```python
from build123d import *

# Parameters (mm, degrees)
F2_W       = 140
F2_H       = 140
F3_DEPTH   = 500
F4_SIZE2   = 100
F4_SIZE    = 40
F4_2_SIZE2 = 100
F4_2_SIZE  = 40
F6_DEPTH   = 70
F7_W       = 60
F7_H       = 40
F8_DEPTH   = 60


with BuildPart() as f3:
    # F2 (on Front) → F3 (new body, symmetric)
    with BuildSketch(Plane.XZ):
        Rectangle(F2_W, F2_H)
    extrude(amount=F3_DEPTH, both=True)

    # F4
    f4_edges = [f3.edges().sort_by_distance(p)[0] for p in [
        (0, -500, 70),
    ]]
    f4_side = f3.faces().sort_by_distance((0, -500, 0))[0]
    chamfer(f4_edges, length=F4_SIZE, length2=F4_SIZE2, reference=f4_side)

    # F4#2
    f4_2_edges = [f3.edges().sort_by_distance(p)[0] for p in [
        (0, 500, 70),
    ]]
    f4_2_side = f3.faces().sort_by_distance((0, 500, 0))[0]
    chamfer(f4_2_edges, length=F4_2_SIZE, length2=F4_2_SIZE2, reference=f4_2_side)

    # F5 (on Right) → F6 (cut, symmetric)
    with BuildSketch(Plane.YZ):
        Polygon((200, -30), (0, -30), (-200, -30), (-300, -70), (0, -70), (300, -70), align=None)
    extrude(amount=F6_DEPTH, both=True, mode=Mode.SUBTRACT)

    # F7 (on face) → F8 (cut)
    with BuildSketch(Plane.XY.offset(70)):
        with Locations((0, -325)):
            Rectangle(F7_W, F7_H)
        with Locations((0, 225)):
            Rectangle(F7_W, F7_H)
    extrude(amount=-F8_DEPTH, mode=Mode.SUBTRACT)


solid = f3.part
```
Design review of the part built by this model. Coordinates are the model's own, in mm. A direction names the side the tool comes from. Coordinates: 2 decimals unless noted, no trailing zeros. Order: outer loops, then holes, each group sorted by start corner. A loop starts at its lowest first (then second) coordinate and runs counter-clockwise, first axis right, second up. Notation, with made-up numbers: M -35.75,75.25 L -20.75,75.25 A22 cw -20.75,92.25 Z; hole C -33.75,88 d1. An arc over 180 degrees is marked long. Answer as a JSON object with one key per item and string values. Group by question number.
1) Wall thickness on L1, parallel to Y at x = -21.5, z = 20; L2, parallel to Z at x = 33, y = 22; L3, parallel to Y at x = -45, z = -59: over which ranges is each line inside the solid? List them lowest first.
2) For pin 1 (3 mm diameter, centred on x = 44.5, z = 51, fed in from +Y); pin 2 (1.5 mm diameter, centred on x = 9, z = 55, fed in from +Y) (3 decimals), all flat-tipped, find the tip position at first contact; note any pin that passes through.
3) Add section D-D, the plane y = 7. Write out the cut boundary in (x, z).
4) Add section B-B, the plane x = -9. Write out the cut boundary in (y, z).
5) Mouldability with a two-part tool opening along X and no side actions: class faces 1 (the flat face through (-30, 225, 40)), 2 (the flat face through (-1, -6, 70)), 3 (the flat face through (30, -325, 40)), 4 (the flat face through (70, -7, -1)) as pulls with the +X half, pulls with the -X half, needs draft (parallel to the pull), parting line crosses it, or undercut.
6) Tool access review of faces 5 (the flat face through (0.98, 250.7, -50.28)), 6 (the flat face through (-1, 500, -19)), 7 (the flat face through (0, 225, 10)): name each direction out of +Z, -Z, +X, -X, +Y, -Y from which nothing blocks a thin tool from reaching the whole face with its end or side.
7) Add section C-C, the plane z = 41.5. Write out the cut boundary in (x, y), then the cut area to 3 significant figures.
8) Add section A-A, the plane z = -55. Write out the cut boundary in (x, y), then the cut area to 3 significant figures.
Computed values:
{
 "1": {"L1": "y = -500 to -345, -305 to 205, 245 to 500", "L2": "z = -30 to 70", "L3": "y = -500 to -272.5, 272.5 to 500"},
 "2": {"pin 1": "stops at y = 451.25", "pin 2": "stops at y = 439.375"},
 "3": {"outline": "M -70,-30 L 70,-30 L 70,70 L -70,70 Z"},
 "4": {"outline": "M -500,-70 L -300,-70 L -200,-30 L 200,-30 L 300,-70 L 500,-70 L 500,30 L 400,70 L 245,70 L 245,10 L 205,10 L 205,70 L -305,70 L -305,10 L -345,10 L -345,70 L -400,70 L -500,30 Z"},
 "5": {"face 1": "undercut", "face 2": "needs draft", "face 3": "undercut", "face 4": "pulls with the +X half"},
 "6": {"face 5": "-Z, +X, -X", "face 6": "+Z, -Z, +X, -X, +Y", "face 7": "+Z"},
 "7": {"outline": "M -70,-471.25 L 70,-471.25 L 70,471.25 L -70,471.25 Z; hole M -30,-345 L 30,-345 L 30,-305 L -30,-305 Z; hole M -30,205 L 30,205 L 30,245 L -30,245 Z", "area": "127,000 mm^2"},
 "8": {"outline": "M -70,-500 L 70,-500 L 70,-262.5 L -70,-262.5 Z; M -70,262.5 L 70,262.5 L 70,500 L -70,500 Z", "area": "66,500 mm^2"}
}
